from build123d import *
from build123d.topology import SkipClean

# Parameters (mm, degrees)
SKETCH1_W                   = 102
SKETCH1_H                   = 102
BOSS_EXTRUDE1_DEPTH         = 50
CUT_EXTRUDE_THIN1_OUTLINE_W = 40
CUT_EXTRUDE_THIN1_OUTLINE_H = 95.773670058
CUT_EXTRUDE_THIN1_DEPTH     = 50
SKETCH4_W                   = 40
SKETCH4_H                   = 6.202657501
CUT_EXTRUDE3_DEPTH          = 54
SKETCH5_W                   = 33.817621941
SKETCH5_H                   = 102.594578927
CUT_EXTRUDE4_DEPTH          = 20
SKETCH6_W                   = 27.820383201
SKETCH6_H                   = 98.886835029
CUT_EXTRUDE5_DEPTH          = 20
SKETCH7_W                   = 30.8
SKETCH7_H                   = 3.364819678
BOSS_EXTRUDE2_DEPTH         = 21
SKETCH9_W                   = 31
SKETCH9_H                   = 3.479961613
BOSS_EXTRUDE4_DEPTH         = 21
SKETCH11_W                  = 98.820383201
SKETCH11_H                  = 3.113164971
BOSS_EXTRUDE6_DEPTH         = 47.625
SKETCH14_W                  = 102
SKETCH14_H                  = 5
CUT_EXTRUDE7_DEPTH          = 105
SKETCH17_R                  = 7
CUT_EXTRUDE12_DEPTH         = 20.5
M3_CLEARANCE_HOLE1_D        = 3.4
SKETCH22_W                  = 3.179616799
SKETCH22_H                  = 102
BOSS_EXTRUDE7_DEPTH         = 47.6
CUT_EXTRUDE13_DEPTH         = 5
CUT_EXTRUDE14_DEPTH         = 5
CUT_EXTRUDE16_DEPTH         = 5


# Read off the part's stored shape, not the designer's step: Cut-Extrude-Thin1
with BuildPart() as part:
    # Sketch1 → Boss-Extrude1 (new body)
    with BuildSketch(Plane(origin=(0, 0, 0), x_dir=(1, 0, 0), z_dir=(0, 1, 0))):
        with Locations((-66.567363259, 25.977216604)):
            Rectangle(SKETCH1_W, SKETCH1_H)
    extrude(amount=BOSS_EXTRUDE1_DEPTH)

    # Sketch2 → Cut-Revolve1 (revolve, cut)
    with SkipClean():  # the faces are left unmerged after this step: merging them gives an invalid solid
        with BuildSketch(Plane(origin=(0, 0, 0), x_dir=(1, 0, 0), z_dir=(0, 1, 0))):
            with BuildLine():
                ThreePointArc((-66.567363259, 73.602216604), (-114.192363259, 25.977216604), (-66.567363259, -21.647783396))
                Line((-66.567363259, -21.647783396), (-66.567363259, 73.602216604))
            make_face()
            with BuildLine():
                Line((-66.567363259, 73.602216604), (-66.567363259, -21.647783396))
                ThreePointArc((-66.567363259, -21.647783396), (-32.891402805, -7.69874385), (-18.942363259, 25.977216604))
                ThreePointArc((-18.942363259, 25.977216604), (-32.891402805, 59.653177058), (-66.567363259, 73.602216604))
            make_face()
        revolve(axis=Axis((-66.567363259, 0, 21.647783396), (0, 0, -1)), mode=Mode.SUBTRACT)
    add(part.part.scale(1), mode=Mode.REPLACE)  # the faces are merged on a copy

    # Cut-Extrude-Thin1 outline → Cut-Extrude-Thin1 (cut)
    with BuildSketch(Plane(origin=(0, 0, 0), x_dir=(1, 0, 0), z_dir=(0, 1, 0))):
        with Locations((-66.567363259, 25.977216604)):
            Rectangle(CUT_EXTRUDE_THIN1_OUTLINE_W, CUT_EXTRUDE_THIN1_OUTLINE_H)
    extrude(amount=CUT_EXTRUDE_THIN1_DEPTH, mode=Mode.SUBTRACT)

    # Sketch4 → Cut-Extrude3 (cut)
    with BuildSketch(Plane(origin=(0, 0, 0), x_dir=(1, 0, 0), z_dir=(0, 1, 0))):
        with Locations((-66.567363259, -25.010947176)):
            Rectangle(SKETCH4_W, SKETCH4_H)
    extrude(amount=CUT_EXTRUDE3_DEPTH, mode=Mode.SUBTRACT)

    # Sketch5 → Cut-Extrude4 (cut)
    with BuildSketch(Plane(origin=(0, 0, 0), x_dir=(1, 0, 0), z_dir=(0, 1, 0))):
        with Locations((-29.658552289, 22.56676217)):
            Rectangle(SKETCH5_W, SKETCH5_H)
    extrude(amount=CUT_EXTRUDE4_DEPTH, mode=Mode.SUBTRACT)

    # Sketch6 → Cut-Extrude5 (cut)
    with BuildSketch(Plane(origin=(0, 0, 0), x_dir=(-1, 0, 0), z_dir=(0, -1, 0))):
        with Locations((100.47755486, 24.420634119)):
            Rectangle(SKETCH6_W, SKETCH6_H)
    extrude(amount=-CUT_EXTRUDE5_DEPTH, mode=Mode.SUBTRACT)

    # Sketch7 → Boss-Extrude2 (add)
    with BuildSketch(Plane(origin=(0, 0, 0), x_dir=(1, 0, 0), z_dir=(0, 1, 0))):
        with Locations((-102.167363259, -23.340373557)):
            Rectangle(SKETCH7_W, SKETCH7_H)
    extrude(amount=BOSS_EXTRUDE2_DEPTH)

    # Sketch9 → Boss-Extrude4 (add)
    with BuildSketch(Plane.XZ.offset(-20)):
        with Locations((-31.067363259, 23.28280259)):
            Rectangle(SKETCH9_W, SKETCH9_H)
    extrude(amount=BOSS_EXTRUDE4_DEPTH)

    # Sketch11 → Boss-Extrude6 (add)
    with BuildSketch(Plane.XZ):
        with Locations((-64.97755486, -75.420634119)):
            Rectangle(SKETCH11_W, SKETCH11_H)
    extrude(amount=BOSS_EXTRUDE6_DEPTH)

    # Sketch14 → Cut-Extrude7 (cut)
    with BuildSketch(Plane(origin=(-15.567363259, 0, 0), x_dir=(0, 0, -1), z_dir=(1, 0, 0))):
        with Locations((25.977216604, 47.5)):
            Rectangle(SKETCH14_W, SKETCH14_H)
    extrude(amount=-CUT_EXTRUDE7_DEPTH, mode=Mode.SUBTRACT)

    # Sketch17 → Cut-Extrude12 (cut)
    with BuildSketch(Plane.XZ.offset(-20)):
        with Locations(Location((-94.167363259, 1.657963718, 0), (0, 0, 270))):
            Circle(SKETCH17_R)
        with Locations(Location((-94.167363259, -53.864051633, 0), (0, 0, 284.685382437))):
            Circle(SKETCH17_R)
        with Locations(Location((-39.167363259, 1.657963718, 0), (0, 0, 349.246729183))):
            Circle(SKETCH17_R)
        with Locations(Location((-39.167363259, -53.864051633, 0), (0, 0, 270))):
            Circle(SKETCH17_R)
    extrude(amount=-CUT_EXTRUDE12_DEPTH, mode=Mode.SUBTRACT)

    # M3 Clearance Hole1 (through all)
    with Locations(Plane(origin=(0, 40.5, 0), x_dir=(-1, 0, 0), z_dir=(0, -1, 0))):
        with Locations((94.167363259, -1.657963718), (39.167363259, -1.657963718), (39.167363259, 53.864051633), (94.167363259, 53.864051633)):
            Hole(M3_CLEARANCE_HOLE1_D / 2)

    # Sketch22 → Boss-Extrude7 (add)
    with BuildSketch(Plane.XZ):
        with Locations((-115.97755486, -25.977216604)):
            Rectangle(SKETCH22_W, SKETCH22_H)
    extrude(amount=BOSS_EXTRUDE7_DEPTH)

    # Sketch23 → Cut-Extrude13 (cut)
    with BuildSketch(Plane.XY.offset(-73.864051633)):
        Polygon((-80.20953571, -41.043521661), (-109.215945966, -41.043521661), (-95.243590197, -15.662912687), (-109.215945966, 8.956478339), (-80.850561351, 8.956478339), (-80.850561351, 3.828273211), (-101.283253659, 3.828273211), (-89.824920325, -16.364034482), (-100.932692761, -36.556342174), (-80.20953571, -36.556342174), align=None)
        Polygon((-26.363381864, -41.043521661), (-55.36979212, -41.043521661), (-41.397436351, -15.662912687), (-55.36979212, 8.956478339), (-27.004407505, 8.956478339), (-27.004407505, 3.828273211), (-47.437099813, 3.828273211), (-35.978766479, -16.364034482), (-47.086538915, -36.556342174), (-26.363381864, -36.556342174), align=None)
    extrude(amount=-CUT_EXTRUDE13_DEPTH, mode=Mode.SUBTRACT)

    # Sketch24 → Cut-Extrude14 (cut)
    with BuildSketch(Plane.XY.offset(-73.864051633)):
        Polygon((-70.742432906, -14.032687035), (-70.742432906, 0.710902709), (-66.255253419, 0.710902709), (-66.255253419, -14.032687035), (-51.511663676, -14.032687035), (-51.511663676, -18.519866522), (-66.255253419, -18.519866522), (-66.255253419, -33.263456266), (-70.742432906, -33.263456266), (-70.742432906, -18.519866522), (-85.48602265, -18.519866522), (-85.48602265, -14.032687035), align=None)
    extrude(amount=-CUT_EXTRUDE14_DEPTH, mode=Mode.SUBTRACT)

    # Sketch25 → Cut-Extrude16 (cut)
    with BuildSketch(Plane.ZY.offset(117.567363259)):
        Polygon((-40.375666466, -41.200782652), (-69.382076723, -41.200782652), (-55.409720954, -15.820173678), (-69.382076723, 8.799217348), (-41.016692107, 8.799217348), (-41.016692107, 3.67101222), (-61.449384415, 3.67101222), (-49.991051082, -16.521295473), (-61.098823518, -36.713603165), (-40.375666466, -36.713603165), align=None)
        Polygon((13.47048738, -41.200782652), (-15.535922877, -41.200782652), (-1.563567107, -15.820173678), (-15.535922877, 8.799217348), (12.829461739, 8.799217348), (12.829461739, 3.67101222), (-7.603230569, 3.67101222), (3.855102764, -16.521295473), (-7.252669672, -36.713603165), (13.47048738, -36.713603165), align=None)
        Polygon((-28.964861623, -13.290621763), (-28.964861623, 1.452967981), (-24.477682136, 1.452967981), (-24.477682136, -13.290621763), (-9.734092392, -13.290621763), (-9.734092392, -17.77780125), (-24.477682136, -17.77780125), (-24.477682136, -32.521390994), (-28.964861623, -32.521390994), (-28.964861623, -17.77780125), (-43.708451366, -17.77780125), (-43.708451366, -13.290621763), align=None)
    extrude(amount=-CUT_EXTRUDE16_DEPTH, mode=Mode.SUBTRACT)


solid = part.part
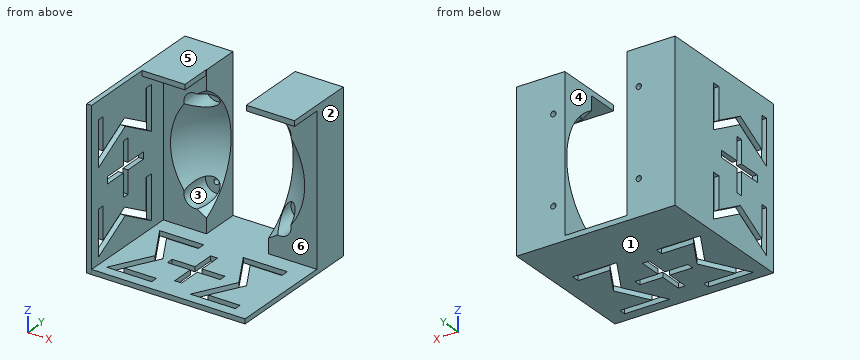
Source: CAD feature listing. Evaluate the final solid. Frame: model axes, mm. Face numbers are marked on the shaded views. A direction names the side the tool comes from. Coordinates: 2 decimals unless noted, no trailing zeros. Loops run counter-clockwise (first coordinate to the right, second up) from the corner with the lowest first, then second, coordinate; pieces in that order, holes last. Notation, with made-up numbers: (-33, 26) -> (-21, 26) arc R26 cw to (-21, 52) -> close; hole circle Ø2 at (17, -13). An arc over 180 degrees is marked (long way). Answer in a Markdown table with one row per item. Add a question column.
Q1. Section B-B on x = -60. Return the cut outline in (y, z) (3 decimals), and give its area (3 significant figures).
Q2. Reachability of the marked faces 4, 5 and 6 from +Z, -Z, +X, -X, +Y, -Y: full face, straight path, thin tool, end or side. Return the list, or none.
Q3. Contact query for flat-ended pins moving along their axis: pin 1 Ø10 at (x, y) = (-62.5, -21) entering from +Z; pin 2 Ø5.5 at (x, z) = (-39.17, -53.86) entering from -Y; pin 3 Ø5 at (x, y) = (-46, -1) entering from -Z. Output: stop coordinate, or through.
Q4. Ray query, line 1 along Z through (x, y) = (-44.5, 18); line 2 along X through (y, z) = (-30, -11); line 3 along Z through (x, y) = (-83, 18.5). Return the intervals inside material, ascending.
Q5. Pull-direction query (X, two-part tool) for the marked faces 1, 2 and 3; classes: pulls with the +X half, pulls with the -X half, needs draft (parallel to the pull), parting line crosses it, or undercut.
Q6. Section C-C on y = -20.5. Give the number of separate pieces and of enclosed holes in the cut face, and give its area (3 significant figures).
Q7. Section A-A on y = 16. Return the cut outline in (x, z), and give its area (3 significant figures).
Computed values:
| question | item | result |
|---|---|---|
| 1 | outline | (-47.625, -76.977) -> (-18.52, -76.977) -> (-18.52, -73.864) -> (-47.625, -73.864) -> close; (-14.033, -76.977) -> (45, -76.977) -> (45, -73.864) -> (-14.033, -73.864) -> close |
| 1 | area | 274 mm^2 |
| 2 | face 4 | +Z, +Y, -Y |
| 2 | face 5 | +Z, +X, -X, +Y, -Y |
| 2 | face 6 | +X, -Y |
| 3 | pin 1 | stops at z = -73.86 |
| 3 | pin 2 | stops at y = 40.5 |
| 3 | pin 3 | stops at z = -76.98 |
| 4 | line 1 | z = -76.98 to -73.86, 21.54 to 25.02 |
| 4 | line 2 | x = -117.57 to -114.39 |
| 4 | line 3 | z = -76.98 to -73.86 |
| 5 | face 1 | needs draft |
| 5 | face 2 | pulls with the +X half |
| 5 | face 3 | undercut |
| 6 | separate pieces | 7 |
| 6 | enclosed holes | 0 |
| 6 | area | 531 mm^2 |
| 7 | outline | (-117.57, -76.98) -> (-15.57, -76.98) -> (-15.57, -73.86) -> (-114.39, -73.86) -> (-114.39, 21.66) -> (-86.77, 21.66) -> (-86.77, 25.02) -> (-117.57, 25.02) -> close; (-46.57, 21.54) -> (-15.57, 21.54) -> (-15.57, 25.02) -> (-46.57, 25.02) -> close |
| 7 | area | 833 mm^2 |
